Check sheet for the modelled part. Datum: model origin and axes. Units: mm. Face numbers are marked on the shaded views. A direction names the side the tool comes from. Round coordinates to 2 decimals unless told otherwise and drop trailing zeros. Order: outer loops, then holes, each group sorted by start corner. A loop starts at its lowest first (then second) coordinate and runs counter-clockwise, first axis right, second up.
Q1. Scan lines: probe 1 along X at (y, z) = (-6.75, 0); probe 2 along X at (y, z) = (0.75, -10); probe 3 along Z at (x, y) = (5, -4.5). Record each from-to range of solid material in increasing order.
Q2. Cross-section at D-D on x = 19. Record the cut outline in (y, z), then the cut area to 3 significant figures.
Q3. Cross-section at A-A on z = 21.5. Record the cut outline in (x, y).
Q4. Mould release check, pull along X, two halves, no side actions. Record for the marked faces 5 and 6: +X half, -X half, draft (parallel to the pull), parting line (faces both ways), or undercut.
Q5. Set-up check for the marked faces 1, 2, 3 and 4: record each of +Z, -Z, +X, -X, +Y, -Y from which the full face is reachable in a straight line by a thin tool's end or side.
Q6. Cross-section at C-C on y = -1.5. Record the cut outline in (x, z), then the cut area to 3 significant figures.
Q7. Cross-section at B-B on x = -9.5. Record the cut outline in (y, z).
Q8. Depth check by flat-ended pin: P1, Ø5, axis at y = 1.5, z = 17.5, coming from the -X side; P2, Ø10, axis at x = 27.5, y = -4.5, coming from the +Z side; P3, Ø10, axis at y = -5.5, z = -11.5, coming from the -X side. Enter the tip coordinate at first touch or a pass-through.
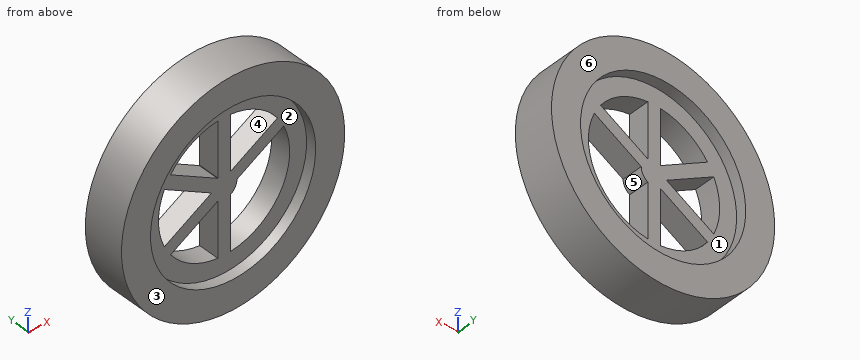
from build123d import *

# Parameters (mm, degrees)
SKETCH1_R           = 53.695322997
BOSS_EXTRUDE2_DEPTH = 10
SKETCH3_R           = 39.733093336
CUT_EXTRUDE2_DEPTH  = 10
SKETCH4_R           = 39.733093336
SKETCH4_R_2         = 31.58457531
BOSS_EXTRUDE3_DEPTH = 5
BOSS_EXTRUDE4_DEPTH = 5
CIRPATTERN3_COUNT   = 5
CIRPATTERN3_ANGLE   = 240


with BuildPart() as part:
    # Sketch1 → Boss-Extrude2 (new, symmetric)
    with BuildSketch(Plane(origin=(0, 0, 0), x_dir=(1, 0, 0), z_dir=(0, 1, 0))):
        with Locations(Location((0, 0, 0), (0, 0, 270))):
            Circle(SKETCH1_R)
    extrude(amount=BOSS_EXTRUDE2_DEPTH, both=True)

    # Sketch3 → Cut-Extrude2 (cut, symmetric)
    with BuildSketch(Plane(origin=(0, 0, 0), x_dir=(1, 0, 0), z_dir=(0, 1, 0))):
        with Locations(Location((0, 0, 0), (0, 0, 270))):
            Circle(SKETCH3_R)
    extrude(amount=CUT_EXTRUDE2_DEPTH, both=True, mode=Mode.SUBTRACT)

    # Sketch4 → Boss-Extrude3 (add, symmetric)
    with BuildSketch(Plane(origin=(0, 0, 0), x_dir=(1, 0, 0), z_dir=(0, 1, 0))):
        with Locations(Location((0, 0, 0), (0, 0, 270))):
            Circle(SKETCH4_R)
        with Locations(Location((0, 0, 0), (0, 0, 270))):
            Circle(SKETCH4_R_2, mode=Mode.SUBTRACT)
    extrude(amount=BOSS_EXTRUDE3_DEPTH, both=True)

    # Sketch6 → Boss-Extrude4 (add, symmetric)
    with BuildSketch(Plane(origin=(0, 0, 0), x_dir=(1, 0, 0), z_dir=(0, 1, 0))):
        with BuildLine():
            Line((3, 5.387115822), (3, 39.619675744))
            Line((3, 39.619675744), (-3, 39.619675744))
            Line((-3, 39.619675744), (-3, 5.387115822))
            ThreePointArc((-3, 5.387115822), (0, -6.166118461), (3, 5.387115822))
        make_face()
    boss_extrude4 = extrude(amount=BOSS_EXTRUDE4_DEPTH, both=True)

    # CirPattern3: Boss-Extrude4 ×5 about axis
    cirpattern3_axis = Axis((0, 0, 0), (0, 1, 0))
    for i in range(1, CIRPATTERN3_COUNT):
        add(boss_extrude4.rotate(cirpattern3_axis, i * CIRPATTERN3_ANGLE / (CIRPATTERN3_COUNT - 1)))


solid = part.part
Results found:
1. probe 1: x = -53.7 to -39.73, 39.73 to 53.7
1. probe 2: x = -52.76 to -29.96, -23.32 to -11.32, -3 to 3, 29.96 to 52.76
1. probe 3: z = -53.46 to -31.19, -3.61 to 6.35, 31.19 to 53.46
2. outline: (-10, -50.22) - (10, -50.22) - (10, -34.9) - (5, -34.9) - (5, -25.23) - (-5, -25.23) - (-5, -34.9) - (-10, -34.9) - close; (-10, 34.9) - (-5, 34.9) - (-5, 25.23) - (5, 25.23) - (5, 34.9) - (10, 34.9) - (10, 50.22) - (-10, 50.22) - close; (-5, 7.51) - (5, 7.51) - (5, 14.43) - (-5, 14.43) - close
2. area: 876 mm2
3. outline: (-49.2, -10) - (-33.41, -10) - (-33.41, -5) - (-23.14, -5) - (-23.14, 5) - (-33.41, 5) - (-33.41, 10) - (-49.2, 10) - close; (-3, -5) - (3, -5) - (3, 5) - (-3, 5) - close; (23.14, -5) - (33.41, -5) - (33.41, -10) - (49.2, -10) - (49.2, 10) - (33.41, 10) - (33.41, 5) - (23.14, 5) - close
4. face 5: undercut
4. face 6: draft
5. face 1: +Y
5. face 2: -Y
5. face 3: +Z, -Z, +X, -X, -Y
5. face 4: +Y, -Y
6. outline: circle Ø107.39 at (0, 0); hole (-28.73, -13.12) - (-6.17, -0.1) arc R6.17 cw to (-6.17, 0.1) - (-28.73, 13.12) arc R31.58 ccw to start; hole (-25.73, -18.32) arc R31.58 ccw to (-3, -31.44) - (-3, -5.39) arc R6.17 cw to (-3.17, -5.29) - close; hole (-25.73, 18.32) - (-3.17, 5.29) arc R6.17 cw to (-3, 5.39) - (-3, 31.44) arc R31.58 ccw to start; hole (3, -31.44) arc R31.58 ccw to (28.73, 13.12) - (6.17, 0.1) arc R6.17 cw to (3, -5.39) - close; hole (3, 5.39) arc R6.17 cw to (3.17, 5.29) - (25.73, 18.32) arc R31.58 ccw to (3, 31.44) - close
6. area: 6,810 mm2
7. outline: (-10, -52.85) - (10, -52.85) - (10, -38.58) - (5, -38.58) - (5, -30.12) - (-5, -30.12) - (-5, -38.58) - (-10, -38.58) - close; (-10, 38.58) - (-5, 38.58) - (-5, 30.12) - (5, 30.12) - (5, 38.58) - (10, 38.58) - (10, 52.85) - (-10, 52.85) - close; (-5, -8.95) - (5, -8.95) - (5, -2.02) - (-5, -2.02) - close; (-5, 2.02) - (5, 2.02) - (5, 8.95) - (-5, 8.95) - close
8. P1: stops at x = -51.56
8. P2: stops at z = 48.75
8. P3: stops at x = -53.3
